Read the model definition and answer for the solid it produces. Units are mm, in the model's axes. A direction names the side the tool comes from. Coordinates: 2 decimals unless noted, no trailing zeros. Loops run counter-clockwise (first coordinate to the right, second up) from the corner with the lowest first, then second, coordinate; pieces in that order, holes last. Notation, with made-up numbers: M 57,75 L 81,75 A7 ccw 81,84 Z; hole C 43.5,29 d9. An arc over 180 degrees is marked long. Put each result on its own line as item: value.
from build123d import *

# Parameters (mm, degrees)
F_01_HOUSING_PROFILE_W        = 60
F_01_HOUSING_PROFILE_H        = 60
F_01_HOUSING_BLOCK_DEPTH      = 560
F_02_FACE_BOSS_PROFILE_R      = 41
F_02_FACE_LOCATING_BOSS_DEPTH = 12


with BuildPart() as part:
    # 01_Housing_Profile → 01_Housing_Block (new body)
    with BuildSketch(Plane(origin=(0, 0, 0), x_dir=(1, 0, 0), z_dir=(0, 1, 0))):
        Rectangle(F_01_HOUSING_PROFILE_W, F_01_HOUSING_PROFILE_H)
    extrude(amount=F_01_HOUSING_BLOCK_DEPTH)

    # 02_Face_Boss_Profile → 02_Face_Locating_Boss (add)
    with BuildSketch(Plane(origin=(0, 0, 0), x_dir=(1, 0, 0), z_dir=(0, 1, 0))):
        Circle(F_02_FACE_BOSS_PROFILE_R)
    extrude(amount=F_02_FACE_LOCATING_BOSS_DEPTH)


solid = part.part
1) Which of the six approach directions +Z, -Z, +X, -X, +Y, -Y give full straight-line access (tool end or side, diameter ignored) to faces 1 (the cylindrical face through (0, 6, -41)), 2 (the flat face through (34, 12, 0)), 3 (the flat face through (-34, 12, 0)), 4 (the flat face through (0, 12, -34)), 5 (the flat face through (0, 12, 34))?
Answer list:
face 1: -Z, +Y, -Y
face 2: +Z, -Z, +X, +Y
face 3: +Z, -Z, -X, +Y
face 4: -Z, +X, -X, +Y
face 5: +Z, +X, -X, +Y
2) Find section D-D, the plane x = 35. Write down the section's boundary in (y, z).
Answer list:
outline: M 0,-21.35 L 12,-21.35 L 12,21.35 L 0,21.35 Z
3) Find section A-A, the plane z = -4.5. Write down the section's boundary in (x, y).
Answer list:
outline: M -40.75,0 L 40.75,0 L 40.75,12 L 30,12 L 30,560 L -30,560 L -30,12 L -40.75,12 Z
4) Find section B-B, the plane x = 8. Write down the section's boundary in (y, z), plus the area to 3 significant figures.
Answer list:
outline: M 0,-40.21 L 12,-40.21 L 12,-30 L 560,-30 L 560,30 L 12,30 L 12,40.21 L 0,40.21 Z
area: 33,800 mm^2
5) Straight lines are drawn through the part: line 1 (X direction, y = 373, z = -15); line 2 (Y direction, x = 34.5, z = -17). For each, find the intervals that lie inside material, in ascending order. Write a range as [from, to].
Answer list:
line 1: x = [-30, 30]
line 2: y = [0, 12]
6) Given pin 1 Ø9 at (x, z) = (11, 35.5) entering from +Y; pin 2 Ø3 at (y, z) = (175.5, -6) entering from -X; pin 3 Ø4 at (x, y) = (-21, 104.5) entering from +Z, each flat-ended and moving along its own axis, determine where each tip first touches the part or whether it passes through.
Answer list:
pin 1: stops at y = 12
pin 2: stops at x = -30
pin 3: stops at z = 30
7) Find section C-C, the plane y = 458. Write down the section's boundary in (x, z).
Answer list:
outline: M -30,-30 L 30,-30 L 30,30 L -30,30 Z
